Build history of the part. All positions in model axes, mm. Coordinates: 2 decimals unless noted, no trailing zeros. Order: outer loops, then holes, each group sorted by start corner. A loop starts at its lowest first (then second) coordinate and runs counter-clockwise, first axis right, second up. Notation, with made-up numbers: (-23, 45) - (18, 45) arc R26 ccw to (18, 81) - close; hole circle Ø2 at (-38.5, 29). An arc over 180 degrees is marked (long way). Return JSON: item names as keys, results as strings.
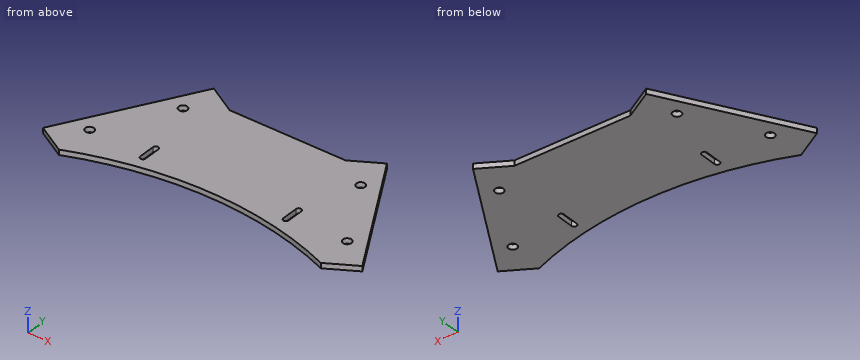
from build123d import *

# Parameters (mm, degrees)
MODEL_R             = 2.6
BOSS_EXTRUDE1_DEPTH = 3.125


with BuildPart() as part:
    # Model → Boss-Extrude1 (new body)
    with BuildSketch(Plane.XY):
        with BuildLine():
            Line((175.590993043, 0), (192.911501119, 10))
            Line((192.911501119, 10), (148.776258635, 86.444482386))
            Line((148.776258635, 86.444482386), (131.455750559, 76.444482386))
            Line((131.455750559, 76.444482386), (61.455750559, 76.444482386))
            Line((61.455750559, 76.444482386), (44.135242484, 86.444482386))
            Line((44.135242484, 86.444482386), (0, 10))
            Line((0, 10), (17.320508076, 0))
            ThreePointArc((17.320508076, 0), (96.455750559, 15.314685), (175.590993043, 0))
        make_face()
        with Locations((42.795496522, 64.123974311)):
            Circle(MODEL_R, mode=Mode.SUBTRACT)
        with Locations((18.660254038, 22.320508076)):
            Circle(MODEL_R, mode=Mode.SUBTRACT)
        with Locations((150.116004597, 64.123974311)):
            Circle(MODEL_R, mode=Mode.SUBTRACT)
        with Locations((174.251247081, 22.320508076)):
            Circle(MODEL_R, mode=Mode.SUBTRACT)
        with BuildLine():
            Line((54.855750559, 29.174833766), (54.855750559, 19.174833766))
            ThreePointArc((54.855750559, 19.174833766), (53.255750559, 17.574833766), (51.655750559, 19.174833766))
            Line((51.655750559, 19.174833766), (51.655750559, 29.174833766))
            ThreePointArc((51.655750559, 29.174833766), (53.255750559, 30.774833766), (54.855750559, 29.174833766))
        make_face(mode=Mode.SUBTRACT)
        with BuildLine():
            Line((141.255750559, 29.174833766), (141.255750559, 19.174833766))
            ThreePointArc((141.255750559, 19.174833766), (139.655750559, 17.574833766), (138.055750559, 19.174833766))
            Line((138.055750559, 19.174833766), (138.055750559, 29.174833766))
            ThreePointArc((138.055750559, 29.174833766), (139.655750559, 30.774833766), (141.255750559, 29.174833766))
        make_face(mode=Mode.SUBTRACT)
    extrude(amount=BOSS_EXTRUDE1_DEPTH)


solid = part.part
1. Cut at B-B on x = 160. Give the cut face in (y, z) (3 decimals).
Check values:
{"outline": "(5.573, 0) - (67.004, 0) - (67.004, 3.125) - (5.573, 3.125) - close"}
2. Drop flat-ended pins along their axis: pin 1 (1.5 mm diameter, centred on y = 11.5, z = 0.5, fed in from +X); pin 2 (1.5 mm diameter, centred on x = 144.5, z = 1, fed in from -Y); pin 3 (7 mm diameter, centred on x = 18.66, y = 22.32, fed in from +Z) (3 decimals); pin 4 (1.5 mm diameter, centred on y = 12.5, z = 0.5, fed in from -X). Give the stop position or say it passes through.
Check values:
{"pin 1": "x = 192.48", "pin 2": "y = 9.63", "pin 3": "z = 3.125", "pin 4": "x = 1.01"}
3. Probe L1, parallel to X at y = 62, z = 1.1; L2, parallel to X at y = 21.5, z = 0.55; L3, parallel to X at y = 40, z = 1.4. List the from-to ranges inside material, lowest first.
Check values:
{"L1": "30.02 to 41.3, 44.3 to 148.62, 151.62 to 162.89", "L2": "6.64 to 16.19, 21.13 to 51.66, 54.86 to 138.06, 141.26 to 171.78, 176.72 to 186.27", "L3": "17.32 to 175.59"}
4. Cut at A-A on z = 1.3. Give the cut face in (x, y).
Check values:
{"outline": "(0, 10) - (17.32, 0) arc R212.11 cw to (175.59, 0) - (192.91, 10) - (148.78, 86.44) - (131.46, 76.44) - (61.46, 76.44) - (44.14, 86.44) - close; hole circle Ø5.2 at (18.66, 22.32); hole circle Ø5.2 at (42.8, 64.12); hole (51.66, 19.17) arc R1.6 ccw to (54.86, 19.17) - (54.86, 29.17) arc R1.6 ccw to (51.66, 29.17) - close; hole (138.06, 19.17) arc R1.6 ccw to (141.26, 19.17) - (141.26, 29.17) arc R1.6 ccw to (138.06, 29.17) - close; hole circle Ø5.2 at (150.12, 64.12); hole circle Ø5.2 at (174.25, 22.32)"}
5. Cut at C-C on y = 56.5. Give the cut face in (x, z) (3 decimals), plus the area to 3 significant figures.
Check values:
{"outline": "(26.847, 0) - (166.065, 0) - (166.065, 3.125) - (26.847, 3.125) - close", "area": "435 mm²"}
